The listing builds one solid part. Answer for the finished solid, in the listing's coordinates (mm). Coordinates: 2 decimals unless noted, no trailing zeros. Write each loop counter-clockwise with the first axis right and the second up, starting at its lowest first coordinate (ties: lowest second). Pieces come first, ordered by that corner, then holes.
from build123d import *

# Parameters (mm, degrees)
SKETCH_1_R          = 72.25
EXTRUDE_7_DEPTH     = 10
F_3_0MM_1_D         = 3
F_3_0MM_1_DEPTH     = 6
F_3_0MM_1_TIP       = 0.901290929
CUT_EXTRUDE_START   = 10
SKETCH_1_11_R       = 71
SKETCH_1_11_R_2     = 68
CUT_EXTRUDE_1_DEPTH = 2


with BuildPart() as part:
    # 草圖1 → 填料-伸長7 (new body)
    with BuildSketch(Plane(origin=(0, 0, 0), x_dir=(1, 0, 0), z_dir=(0, 1, 0))):
        with Locations(Location((0, 0, 0), (0, 0, 270))):
            Circle(SKETCH_1_R)
    extrude(amount=EXTRUDE_7_DEPTH)

    # Ø3.0mm 定位孔1
    with Locations(Plane(origin=(0, 10, 0), x_dir=(1, 0, 0), z_dir=(0, 1, 0))):
        with Locations((-30, 30), (-30, -30), (30, -30), (30, 30)):
            Hole(F_3_0MM_1_D / 2, depth=F_3_0MM_1_DEPTH)
            with Locations((0, 0, -(F_3_0MM_1_DEPTH + F_3_0MM_1_TIP / 2))):  # 118° drill point
                Cone(0, F_3_0MM_1_D / 2, F_3_0MM_1_TIP, mode=Mode.SUBTRACT)

    # 草圖1<11> → 除料-伸長1 (cut)
    with BuildSketch(Plane(origin=(0, 0, 0), x_dir=(1, 0, 0), z_dir=(0, 1, 0)).offset(CUT_EXTRUDE_START)):
        with Locations(Location((0, 0, 0), (0, 0, 270))):
            Circle(SKETCH_1_11_R)
        with Locations(Location((0, 0, 0), (0, 0, 270))):
            Circle(SKETCH_1_11_R_2, mode=Mode.SUBTRACT)
    extrude(amount=-CUT_EXTRUDE_1_DEPTH, mode=Mode.SUBTRACT)


solid = part.part
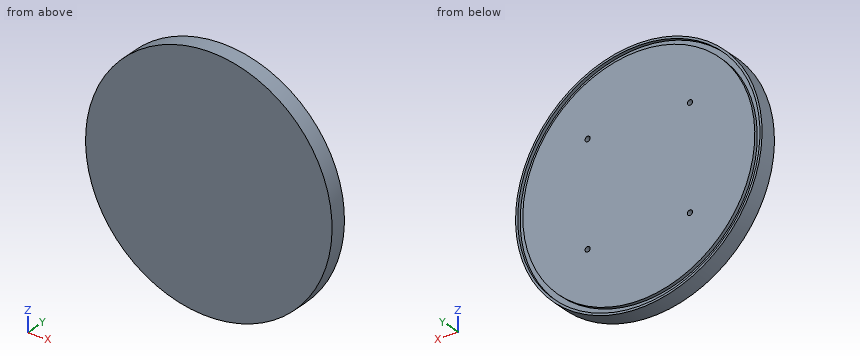
1. Section A-A on x = 44 is taken. Give the vertices of the cut face in (y, z), then the cut area to 3 significant figures.
Results found:
outline: (0, -57.31) - (10, -57.31) - (10, -55.72) - (8, -55.72) - (8, -51.85) - (10, -51.85) - (10, 51.85) - (8, 51.85) - (8, 55.72) - (10, 55.72) - (10, 57.31) - (0, 57.31) - close
area: 1,130 mm2
2. Find the intervals of material crossed by L1, parallel to X at y = 8.6, z = 0; L2, parallel to X at y = 5.65, z = 30, in increasing order.
Results found:
L1: x = -72.25 to -71, -68 to 68, 71 to 72.25
L2: x = -65.73 to -31.5, -28.5 to 28.5, 31.5 to 65.73
3. Section B-B on z = -17.5 is taken. Give the vertices of the cut face in (x, y), then the cut area to 3 significant figures.
Results found:
outline: (-70.1, 0) - (70.1, 0) - (70.1, 10) - (68.81, 10) - (68.81, 8) - (65.71, 8) - (65.71, 10) - (-65.71, 10) - (-65.71, 8) - (-68.81, 8) - (-68.81, 10) - (-70.1, 10) - close
area: 1,390 mm2
4. Flat-ended cylindrical pins translate along their axes: P1, Ø5, axis at x = -30, z = -30, coming from the -Y side; P2, Ø2, axis at y = 1.5, z = 33.5, coming from the -X side; P3, Ø1, axis at x = 10, y = 8.5, coming from the +Z side; P4, Ø2, axis at y = 1.5, z = -4.5, coming from the +X side. Find the tip coordinate at first contact, or state that the pin passes through.
Results found:
P1: stops at y = 0
P2: stops at x = -64.53
P3: stops at z = 71.62
P4: stops at x = 72.17
